Source: CAD feature listing. Evaluate the final solid. Frame: model axes, mm. Round coordinates to 2 decimals unless told otherwise and drop trailing zeros. One line per question, with ' | ' between items.
Autodesk Inventor part; units mm, degrees
ref_plane "YZ Plane" through (0, 0, 0) normal (1, 0, 0) x (0, 1, 0)
ref_plane "XZ Plane" through (0, 0, 0) normal (0, 1, 0) x (-1, 0, 0)
ref_plane "XY Plane" through (0, 0, 0) normal (0, 0, 1) x (1, 0, 0)
sketch "Sketch1" plane through (0, 0, 0) normal (0, 0, 1) x (1, 0, 0)
  line L0 (15.9308, -18.6059) -> (-31.3132, -18.6059)
  line L1 (-31.3132, -18.6059) -> (-31.3132, 20.3831)
  line L2 (-31.3132, 20.3831) -> (15.9308, 20.3831)
  line L3 (15.9308, 20.3831) -> (15.9308, -18.6059)
  point P0 (0, 0)
  dimension "d0" = 38.989
  dimension "d1" = 47.244
extrude "Extrusion1" add sketch "Sketch1" along normal blind 1.67
sketch "Sketch2" plane through (0, 0, 1.67) normal (0, 0, 1) x (1, 0, 0)
  line L0 (-31.3132, -18.6059) -> (15.9308, -18.6059)
  line L1 (15.9308, -18.6059) -> (15.9308, 20.3831)
  line L2 (15.9308, 20.3831) -> (-31.3132, 20.3831)
  line L3 (-31.3132, 20.3831) -> (-31.3132, -18.6059)
  circle A0 centre (-28.1382, 14.0331) radius 0.7937
  circle A1 centre (12.7558, 14.0331) radius 0.7937
  circle A2 centre (12.7558, -2.7309) radius 0.7937
  circle A3 centre (-28.1382, -2.7309) radius 0.7937
  point P0 (0, 0)
  dimension "d4" = 1.5875
  dimension "d5" = 1.5875
  dimension "d6" = 1.5875
  dimension "d7" = 1.5875
  dimension "d8" = 3.175
  dimension "d9" = 3.175
  dimension "d10" = 3.175
  dimension "d11" = 3.175
  dimension "d12" = 15.875
  dimension "d13" = 15.875
  dimension "d14" = 6.35
  dimension "d15" = 6.35
extrude "Extrusion2" cut sketch "Sketch2" against normal up to next contours A0 | A1 | A2 | A3
properties part number "CombinerBoard"
1. Contact query for a flat-ended pin moving along its axis: P1, Ø1, axis at x = 3.5, y = 3, coming from the -Z side. Output: stop coordinate, or through.
Worked out:
P1: stops at z = 0
2. Material intervals for probe 1 along Y at (x, z) = (-28, 1.45); probe 2 along X at (y, z) = (14, 1.2); probe 3 along X at (y, z) = (-2.5, 0.85), sorted ascending.
Worked out:
probe 1: y = -18.61 to -3.51, -1.95 to 13.25, 14.81 to 20.38 | probe 2: x = -31.31 to -28.93, -27.35 to 11.96, 13.55 to 15.93 | probe 3: x = -31.31 to -28.9, -27.38 to 12, 13.52 to 15.93
3. Mould query, pull axis Y, two halves, no side actions, for faces 1 (the cylindrical face through (11.963, -2.696, 0.847)), 2 (the flat face through (-7, -18.606, 1)), 3 (the flat face through (-31.313, 1, 1)). Classes: released by +Y, released by -Y, zero draft, split by the parting line, or undercut.
Worked out:
face 1: undercut | face 2: released by -Y | face 3: zero draft
